Input: part model. Units: mm. Frame: model coordinates. Face numbers are marked on the shaded views. A direction names the side the tool comes from. Coordinates: 2 decimals unless noted, no trailing zeros. Loops run counter-clockwise (first coordinate to the right, second up) from the corner with the lowest first, then second, coordinate; pieces in that order, holes last. Notation, with made-up numbers: (-23.5, -6) - (11.5, -6) arc R24 cw to (11.5, 9) - close; hole circle Ø5 at (50, 13.25). An arc over 180 degrees is marked (long way). Use a Markdown table: item, result. Add a question column.
1. Contact query for flat-ended pins moving along their axis: P1, Ø6, axis at x = 4, z = -5.5, coming from the -Y side; P2, Ø1.9, axis at x = 12.5, y = 18, coming from the +Z side; P3, Ø4.5, axis at x = 10, z = 0, coming from the -Y side. Output: stop coordinate, or through.
2. Section query C-C on z = 6. Return the cut outline in (x, y), then the cut area to 3 significant figures.
3. Ray query, L1, parallel to Y at x = 10, z = 5.5; L2, parallel to Y at x = 10, z = 3.5; L3, parallel to Z at x = 14.75, y = 17. Return the intervals inside material, ascending. Write a range as [from, to].
4. Section query A-A on x = 2.75. Return the cut outline in (y, z), then the cut area to 3 significant figures.
5. Access query for the marked faces 1 and 2. Directions: +Z, -Z, +X, -X, +Y, -Y. A direction counts if a zero-diameter tool reaches every point of the face in a straight line with its end or side. Return the directions, or none.
6. Draft query along X for the marked faces 3, 4 and 5. Return one class per face: released by +X, released by -X, zero draft, split by the parting line, or undercut.
7. Section query D-D on z = 0. Return the cut outline in (x, y).
8. Section query B-B on y = 17. Return the cut outline in (x, z).
```python
from build123d import *

# Parameters (mm, degrees)
SKETCH_1_R          = 3
EXTRUDE_1_DEPTH     = 8
EXTRUDE_1_2_DEPTH   = 8
SKETCH_1_3_R        = 17
SKETCH_1_3_R_2      = 8
EXTRUDE_2_DEPTH     = 20
EXTRUDE_3_REACH     = 39
SKETCH_2_W          = 20
SKETCH_2_H          = 20
SKETCH_3_W          = 20
SKETCH_3_H          = 2
CUT_EXTRUDE_1_DEPTH = 20
SKETCH_4_R          = 2.5
CUT_EXTRUDE_2_DEPTH = 41
SKETCH_5_R          = 2.5
CUT_EXTRUDE_3_DEPTH = 18


with BuildPart() as part:
    # Sketch 1 → Extrude 1 (new body)
    with BuildSketch(Plane(origin=(0, 0, 0), x_dir=(0, 0, -1), z_dir=(1, 0, 0))):
        with BuildLine():
            Line((-7.18451045, 15.40723238), (-30, 4.768194878))
            Line((-30, 4.768194878), (-30, -4.768194878))
            Line((-30, -4.768194878), (-7.18451045, -15.40723238))
            ThreePointArc((-7.18451045, -15.40723238), (-17, 0), (-7.18451045, 15.40723238))
        make_face()
        with Locations((-24, 0)):
            Circle(SKETCH_1_R, mode=Mode.SUBTRACT)
    extrude(amount=EXTRUDE_1_DEPTH)



with BuildPart() as body_2:
    # Sketch 1 → Extrude 1 2 (new body)
    with BuildSketch(Plane(origin=(0, 0, 0), x_dir=(0, 0, -1), z_dir=(1, 0, 0))):
        with BuildLine():
            Line((30, 4.768194878), (7.18451045, 15.40723238))
            ThreePointArc((7.18451045, 15.40723238), (14.337654579, 9.134093342), (17, 0))
            ThreePointArc((17, 0), (14.337654579, -9.134093342), (7.18451045, -15.40723238))
            Line((7.18451045, -15.40723238), (30, -4.768194878))
            Line((30, -4.768194878), (30, 4.768194878))
        make_face()
        with Locations((24, 0)):
            Circle(SKETCH_1_R, mode=Mode.SUBTRACT)
    extrude(amount=EXTRUDE_1_2_DEPTH)


with BuildPart() as part_1:
    add(part.part)

    add(body_2.part)  # Extrude 2 merges body 2
    # Sketch 1_3 → Extrude 2 (add)
    with BuildSketch(Plane(origin=(0, 0, 0), x_dir=(0, 0, -1), z_dir=(1, 0, 0))):
        Circle(SKETCH_1_3_R)
        Circle(SKETCH_1_3_R_2, mode=Mode.SUBTRACT)
    extrude(amount=EXTRUDE_2_DEPTH)

    # Sketch 2 → Extrude 3 (add, up to next)
    with BuildSketch(Plane(origin=(0, 20, 0), x_dir=(1, 0, 0), z_dir=(0, 1, 0)), mode=Mode.PRIVATE) as extrude_3_sk1:
        with Locations((10, 0)):
            Rectangle(SKETCH_2_W, SKETCH_2_H)
    extrude_3_tool1 = extrude(extrude_3_sk1.sketch, amount=-EXTRUDE_3_REACH, mode=Mode.PRIVATE) - part_1.part
    add(extrude_3_tool1.solids().sort_by_distance((10, 20, 0))[0])

    # Sketch 3 → Cut-Extrude 1 (cut)
    with BuildSketch(Plane(origin=(0, 20, 0), x_dir=(1, 0, 0), z_dir=(0, 1, 0))):
        with Locations((10, 0)):
            Rectangle(SKETCH_3_W, SKETCH_3_H)
    extrude(amount=-CUT_EXTRUDE_1_DEPTH, mode=Mode.SUBTRACT)

    # Sketch 4 → Cut-Extrude 2 (cut, through all)
    with BuildSketch(Plane.XY.offset(10)):
        with Locations((10, 17)):
            Circle(SKETCH_4_R)
    extrude(amount=-CUT_EXTRUDE_2_DEPTH, mode=Mode.SUBTRACT)

    # Sketch 5 → Cut-Extrude 3 (cut, through all)
    with BuildSketch(Plane(origin=(0, 0, 0), x_dir=(1, 0, 0), z_dir=(0, 1, 0))):
        with Locations((10, 0)):
            Circle(SKETCH_5_R)
    extrude(amount=-CUT_EXTRUDE_3_DEPTH, mode=Mode.SUBTRACT)


solid = part_1.part
```
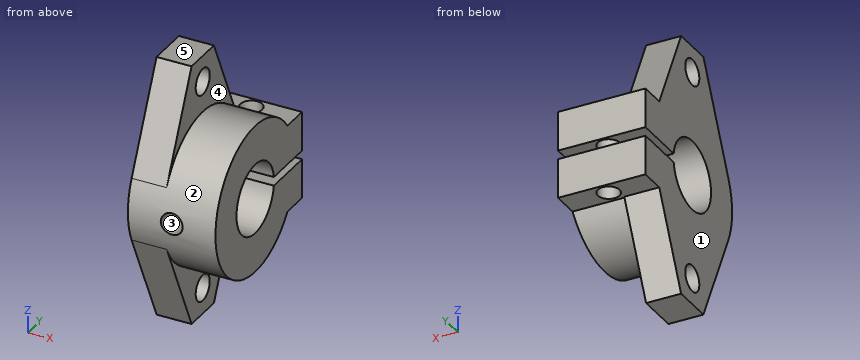
Resolved:
| question | item | result |
|---|---|---|
| 1 | P1 | y = -16.82 |
| 1 | P2 | z = 10 |
| 1 | P3 | y = 7.68 |
| 2 | outline | (0, -15.91) - (20, -15.91) - (20, -5.29) - (0, -5.29) - close; (0, 5.29) - (20, 5.29) - (20, 20) - (0, 20) - close; hole circle Ø5 at (10, 17) |
| 2 | area | 487 mm² |
| 3 | L1 | [-16.09, -5.81], [5.81, 14.5], [19.5, 20] |
| 3 | L2 | [-16.64, -7.19], [7.19, 14.5], [19.5, 20] |
| 3 | L3 | [-10, -1], [1, 10] |
| 4 | outline | (-15.41, -7.18) - (-4.77, -30) - (4.77, -30) - (14.09, -10) - (20, -10) - (20, -1) - (7.94, -1) arc R8 cw (long way) to (7.94, 1) - (20, 1) - (20, 10) - (14.09, 10) - (4.77, 30) - (-4.77, 30) - (-15.41, 7.18) arc R17 ccw to start; hole circle Ø6 at (0, -24); hole circle Ø6 at (0, 24) |
| 4 | area | 1,190 mm² |
| 5 | face 1 | +Z, -Z, -X, +Y, -Y |
| 5 | face 2 | +X |
| 6 | face 3 | undercut |
| 6 | face 4 | released by +X |
| 6 | face 5 | zero draft |
| 7 | outline | (0, -17) - (7.5, -17) - (7.5, -8) - (0, -8) - close; (12.5, -17) - (20, -17) - (20, -8) - (12.5, -8) - close |
| 8 | outline | (0, -10) - (7.5, -10) - (7.5, -1) - (0, -1) - close; (0, 1) - (7.5, 1) - (7.5, 10) - (0, 10) - close; (12.5, -10) - (20, -10) - (20, -1) - (12.5, -1) - close; (12.5, 1) - (20, 1) - (20, 10) - (12.5, 10) - close |
